Here's how the part is built. I have some questions about the finished solid (model axes, mm). Face numbers are marked on the shaded views. Round coordinates to 2 decimals unless told otherwise and drop trailing zeros. Loops run counter-clockwise (first coordinate to the right, second up) from the corner with the lowest first, then second, coordinate; pieces in that order, holes last. Notation, with made-up numbers: M -35,-38 L 0,-38 A34 ccw 0,-3 Z; hole C 48.5,-23.75 d2. An arc over 180 degrees is marked long. Write each question's results on one line, items separated by ' | '. Start each with the question number.
Autodesk Inventor part; units mm, degrees
ref_plane "YZ Plane" through (0, 0, 0) normal (1, 0, 0) x (0, 1, 0)
ref_plane "XZ Plane" through (0, 0, 0) normal (0, 1, 0) x (-1, 0, 0)
ref_plane "XY Plane" through (0, 0, 0) normal (0, 0, 1) x (1, 0, 0)
sketch "スケッチ2" plane through (0, 0, 0) normal (0, 0, 1) x (1, 0, 0)
  circle A0 centre (0, 0) radius 15.8
  dimension "d0" = 31.6
extrude "押し出し1" add sketch "スケッチ2" against normal blind 5
sketch "スケッチ3" plane through (0, 0, 0) normal (0, 0, 1) x (1, 0, 0)
  line L0 (0, 0) -> (0, 20.2537) construction
  circle A0 centre (0, -3) radius 1.7
  circle A1 centre (-10, -6) radius 1.7
  circle A2 centre (10, -6) radius 1.7
  dimension "d32" = 3.4
  dimension "d33" = 3
  dimension "d67" = 3.4
  dimension "d68" = 3.4
  dimension "d69" = 10
  dimension "d70" = 6
extrude "押し出し2" cut sketch "スケッチ3" against normal through all
sketch "スケッチ10" plane through (0, 0, 0) normal (0, 0, 1) x (1, 0, 0)
  circle A0 centre (0, -11.5) radius 1.5
  circle A1 centre (9.9593, 5.75) radius 1.5
  circle A2 centre (-9.9593, 5.75) radius 1.5
  point P0 (0, 0)
  dimension "d71" = 3
  dimension "d72" = 11.5
  dimension "d75" = 360
extrude "押し出し8" cut sketch "スケッチ10" against normal through all
thread "ねじ6"
thread "ねじ7"
thread "ねじ8"
properties part number "B_pipe_cylinder_5" material "ステンレス鋼 440C"
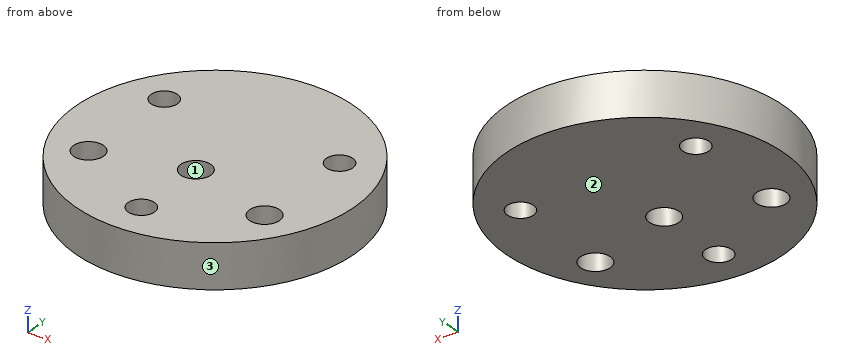
1. For pin 1 (2 mm diameter, centred on x = 10, y = -6, fed in from +Z); pin 2 (1.5 mm diameter, centred on y = -6, z = -1, fed in from +X); pin 3 (3 mm diameter, centred on y = -12.5, z = -1, fed in from +X), each with a flat end and sliding along its axis, tell me the tip position at first contact or that it passes through.
2. If we mould it in two halves opening along X, with no side actions, what happens to the marked faces 1, 2 and 3? For each: released by +X, released by -X, zero draft, split by the parting line, or undercut.
3. I want a section at C-C on x = -10. List the corners of the cut face in (y, z) for me.
4. I need wall thicknesses on line 1 along Y through (x, z) = (0, -3.65); line 2 along Y through (x, z) = (10, -3.55); line 3 along X through (y, z) = (-7.5, -2.6). Which ranges of each line are inside material? Lowest first, please.
5. I want a section at D-D on y = -7. List the corners of the cut face in (x, z) for me, plus the area to 3 significant figures.
6. I want a section at B-B on y = -11.5. List the corners of the cut face in (x, z) for me.
7. I want a section at A-A on z = -4.4. List the corners of the cut face in (x, y) for me.
Outcome:
1) pin 1: through | pin 2: x = 14.9 | pin 3: x = 11.34
2) face 1: undercut | face 2: zero draft | face 3: split by the parting line
3) outline: M -12.23,-5 L -7.7,-5 L -7.7,0 L -12.23,0 Z; M -4.3,-5 L 4.25,-5 L 4.25,0 L -4.3,0 Z; M 7.25,-5 L 12.23,-5 L 12.23,0 L 7.25,0 Z
4) line 1: -15.8 to -13, -10 to -4.7, -1.3 to 15.8 | line 2: -12.23 to -7.7, -4.3 to 4.25, 7.25 to 12.23 | line 3: -13.91 to -10.8, -9.2 to 9.2, 10.8 to 13.91
5) outline: M -14.16,-5 L -11.37,-5 L -11.37,0 L -14.16,0 Z; M -8.63,-5 L 8.63,-5 L 8.63,0 L -8.63,0 Z; M 11.37,-5 L 14.16,-5 L 14.16,0 L 11.37,0 Z | area: 114 mm2
6) outline: M -10.83,-5 L -1.5,-5 L -1.5,0 L -10.83,0 Z; M 1.5,-5 L 10.83,-5 L 10.83,0 L 1.5,0 Z
7) outline: C 0,0 d31.6; hole C -10,-6 d3.4; hole C -9.96,5.75 d3; hole C 0,-3 d3.4; hole C 0,-11.5 d3; hole C 10,-6 d3.4; hole C 9.96,5.75 d3
